The listing builds one solid part. Answer for the finished solid, in the listing's coordinates (mm). Give positions to 0.01 mm unless a question says otherwise; leave off trailing zeros. Order: outer loops, then holes, each group sorted by start corner. A loop starts at its lowest first (then second) coordinate and runs counter-clockwise, first axis right, second up. Notation, with made-up numbers: (15, 2) - (31, 2) arc R34 cw to (31, 32) - close; hole circle Ø5 at (49.5, 83.25). An arc over 180 degrees is marked (long way). Write each question's results on one line, items separated by ' | '. Start each with the question number.
1. Section C-C (x = -16.5) is taken. Give the vertices of the cut face in (y, z), and give its area (3 significant figures).
2. Section A-A (x = -368) is taken. Give the vertices of the cut face in (y, z).
3. Section B-B (z = 5.25) is taken. State how many separate pieces and enclosed holes the cut face has, and give its area (3 significant figures).
4. Flat-ended cylindrical pins translate along their axes: pin 1 (3 mm diameter, centred on x = -217.39, y = 12.85, fed in from +Z); pin 2 (2.5 mm diameter, centred on y = 42.5, z = 3, fed in from +X); pin 3 (13.5 mm diameter, centred on x = -254.48, y = 1.85, fed in from +Z); pin 4 (2.5 mm diameter, centred on y = -32.5, z = 2.5, fed in from -X). Find the tip coordinate at first contact, or state that the pin passes through.
5. Find the intervals of material crossed by L1, parallel to Y at x = -352.5, z = 1.5; L2, parallel to X at y = 0, z = 1.5; L3, parallel to X at y = 30, z = 5.25, in increasing order.
from build123d import *

# Parameters (mm, degrees)
ESQUISSE1_R             = 1.55
BOSS_EXTRU_1_DEPTH      = 8
ESQUISSE2_W             = 508.684044726
ESQUISSE2_H             = 12
ENL_V_MAT_EXTRU_1_DEPTH = 4
ESQUISSE3_R             = 7.5
ENL_V_MAT_EXTRU_2_DEPTH = 10
ESQUISSE4_W             = 101
ESQUISSE4_H             = 60.6
ENL_V_MAT_EXTRU_3_DEPTH = 4
ESQUISSE5_R             = 1
ENL_V_MAT_EXTRU_4_DEPTH = 4


with BuildPart() as part:
    # Esquisse1 → Boss.-Extru.1 (new body)
    with BuildSketch(Plane.XY):
        with BuildLine():
            Line((-399.388568491, 52.350857253), (-399.388568491, 24.472177597))
            ThreePointArc((-399.388568491, 24.472177597), (-399.388568491, 22.350857253), (-401.509888834, 22.350857253))
            Line((-401.509888834, 22.350857253), (-407.388568491, 22.350857253))
            Line((-407.388568491, 22.350857253), (-407.388568491, -17.649142747))
            Line((-407.388568491, -17.649142747), (-401.509888834, -17.649142747))
            ThreePointArc((-401.509888834, -17.649142747), (-399.388568491, -17.649142747), (-399.388568491, -19.77046309))
            Line((-399.388568491, -19.77046309), (-399.388568491, -47.649142747))
            Line((-399.388568491, -47.649142747), (84.611431509, -47.649142747))
            Line((84.611431509, -47.649142747), (84.611431509, -19.77046309))
            ThreePointArc((84.611431509, -19.77046309), (84.611431509, -17.649142747), (86.732751853, -17.649142747))
            Line((86.732751853, -17.649142747), (92.611431509, -17.649142747))
            Line((92.611431509, -17.649142747), (92.611431509, 22.350857253))
            Line((92.611431509, 22.350857253), (86.732751853, 22.350857253))
            ThreePointArc((86.732751853, 22.350857253), (84.611431509, 22.350857253), (84.611431509, 24.472177597))
            Line((84.611431509, 24.472177597), (84.611431509, 52.350857253))
            Line((84.611431509, 52.350857253), (-399.388568491, 52.350857253))
        make_face()
        with Locations((-403.388568491, 2.350857253)):
            Circle(ESQUISSE1_R, mode=Mode.SUBTRACT)
        with Locations(Location((88.611431509, 2.350857253, 0), (0, 0, 180))):
            Circle(ESQUISSE1_R, mode=Mode.SUBTRACT)
    extrude(amount=BOSS_EXTRU_1_DEPTH)

    # Esquisse2 → Enlèv. mat.-Extru.1 (cut)
    with BuildSketch(Plane.XY.offset(8)):
        with Locations((-159.986239331, 46.350857253)):
            Rectangle(ESQUISSE2_W, ESQUISSE2_H)
    extrude(amount=-ENL_V_MAT_EXTRU_1_DEPTH, mode=Mode.SUBTRACT)

    # Esquisse3 → Enlèv. mat.-Extru.2 (cut)
    with BuildSketch(Plane.XY.offset(8)):
        with Locations((-254.476180512, 1.850857253)):
            Circle(ESQUISSE3_R)
        with BuildLine():
            Line((-374.489430688, -14.649142747), (-285.287706293, -14.649142747))
            ThreePointArc((-285.287706293, -14.649142747), (-282.388568491, -14.649142747), (-282.388568491, -11.750004944))
            Line((-282.388568491, -11.750004944), (-282.388568491, 15.45171945))
            ThreePointArc((-282.388568491, 15.45171945), (-282.388568491, 18.350857253), (-285.287706293, 18.350857253))
            Line((-285.287706293, 18.350857253), (-374.489430688, 18.350857253))
            ThreePointArc((-374.489430688, 18.350857253), (-377.388568491, 18.350857253), (-377.388568491, 15.45171945))
            Line((-377.388568491, 15.45171945), (-377.388568491, -11.750004944))
            ThreePointArc((-377.388568491, -11.750004944), (-377.388568491, -14.649142747), (-374.489430688, -14.649142747))
        make_face()
    extrude(amount=-ENL_V_MAT_EXTRU_2_DEPTH, mode=Mode.SUBTRACT)

    # Esquisse4 → Enlèv. mat.-Extru.3 (cut)
    with BuildSketch(Plane.XY.offset(8)):
        with Locations((-329.888568491, 1.350857253)):
            Rectangle(ESQUISSE4_W, ESQUISSE4_H)
    extrude(amount=-ENL_V_MAT_EXTRU_3_DEPTH, mode=Mode.SUBTRACT)

    # Esquisse5 → Enlèv. mat.-Extru.4 (cut)
    with BuildSketch(Plane.XY.offset(8)):
        with Locations((-263.388568491, -9.149142747)):
            Circle(ESQUISSE5_R)
        with Locations(Location((-263.388568491, 12.850857253, 0), (0, 0, 180))):
            Circle(ESQUISSE5_R)
        with Locations((-217.388568491, 12.850857253)):
            Circle(ESQUISSE5_R)
        with Locations(Location((-217.388568491, -9.149142747, 0), (0, 0, 180))):
            Circle(ESQUISSE5_R)
        with Locations((-204.388008491, 17.350757253)):
            Circle(ESQUISSE5_R)
        with Locations((-182.389068491, 17.350757253)):
            Circle(ESQUISSE5_R)
        with Locations((-204.388008491, -28.648642747)):
            Circle(ESQUISSE5_R)
        with Locations((-182.389068491, -28.648642747)):
            Circle(ESQUISSE5_R)
    extrude(amount=-ENL_V_MAT_EXTRU_4_DEPTH, mode=Mode.SUBTRACT)


solid = part.part
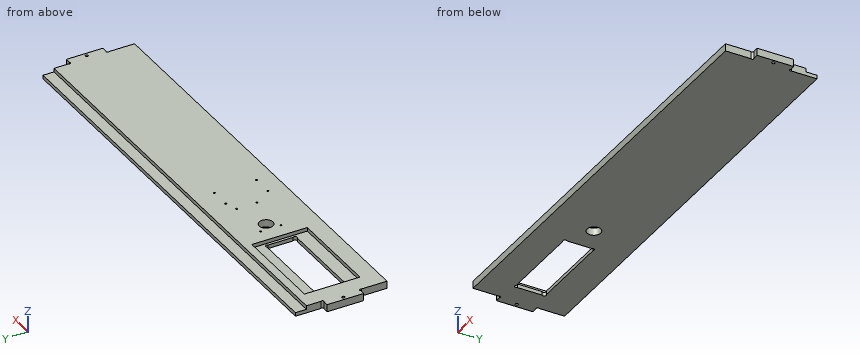
Reported:
1) outline: (-47.65, 0) - (52.35, 0) - (52.35, 4) - (40.35, 4) - (40.35, 8) - (-47.65, 8) - close | area: 752 mm²
2) outline: (-47.65, 0) - (-14.65, 0) - (-14.65, 4) - (-28.95, 4) - (-28.95, 8) - (-47.65, 8) - close; (18.35, 0) - (52.35, 0) - (52.35, 4) - (40.35, 4) - (40.35, 8) - (31.65, 8) - (31.65, 4) - (18.35, 4) - close
3) separate pieces: 1 | enclosed holes: 12 | area: 36,900 mm²
4) pin 1: z = 8 | pin 2: x = 84.61 | pin 3: through | pin 4: x = -399.39
5) L1: -47.65 to -14.65, 18.35 to 52.35 | L2: -407.39 to -377.39, -282.39 to -261.74, -247.21 to 92.61 | L3: -399.39 to -380.39, -279.39 to 84.61
